Autodesk Inventor part; units mm, degrees
ref_plane "YZ Plane" through (0, 0, 0) normal (1, 0, 0) x (0, 1, 0)
ref_plane "XZ Plane" through (0, 0, 0) normal (0, 1, 0) x (-1, 0, 0)
ref_plane "XY Plane" through (0, 0, 0) normal (0, 0, 1) x (1, 0, 0)
sketch "Esboço1" plane through (0, 0, 0) normal (0, 1, 0) x (-1, 0, 0)
  circle A0 centre (0, 0) radius 9
  dimension "d0" = 18
extrude "Extrusão1" add sketch "Esboço1" along normal blind 5
sketch "Esboço2" plane through (0, 5, 0) normal (0, 1, 0) x (1, 0, 0)
  circle A0 centre (0, 0) radius 6
  dimension "d3" = 12
extrude "Extrusão2" add sketch "Esboço2" along normal blind 15
sketch "Esboço3" plane through (0, 20, 0) normal (0, 1, 0) x (1, 0, 0)
  point P0 (0, 0)
sketch "Esboço4" plane through (0, 20, 0) normal (0, 1, 0) x (1, 0, 0)
  circle A0 centre (0, 0) radius 4.275
  dimension "d6" = 8.55
extrude "Extrusão3" cut sketch "Esboço4" against normal through all
fillet "Arredondamento1" radius 2 1 edges at (-6, 5, 0)
properties part number "Espaçadores"
The model under review builds one solid part; all positions refer to its coordinate system, in mm. A direction names the side the tool comes from. Give positions to 0.01 mm unless a question says otherwise; leave off trailing zeros. Write each loop counter-clockwise with the first axis right and the second up, starting at its lowest first coordinate (ties: lowest second). Pieces come first, ordered by that corner, then holes. Notation, with made-up numbers: M 45.25,49 L 78.25,49 A19 cw 78.25,83 Z; hole C -36.75,-21.5 d3. An arc over 180 degrees is marked long. Write item = value, one per line. Start each with the question number.
Q1. For line 1 (Z direction, x = 0, y = 9.75) (3 decimals); line 2 (Z direction, x = 2, y = 15.25), list the stretches that pass through material, from the lowest coordinate up.
Q2. We need section C-C (y = 4.5). State the section outline as (x, z) points (3 decimals).
Q3. We need section A-A (z = 0). State the section outline as (x, y) points (3 decimals).
Q4. We need section B-B (x = 0). State the section outline as (y, z) points (3 decimals), plus the area to 3 significant figures.
Q5. Clearance check with flat-ended pins moving along their axes: pin 1 (4 mm diameter, centred on x = -5.5, y = 6, fed in from -Z); pin 2 (6 mm diameter, centred on y = 16, z = -6.5, fed in from -X); pin 3 (4 mm diameter, centred on x = -4, y = 6.5, fed in from +Z). State where each tip first meets the part, or that it passes through.
Q6. Mouldability with a two-part tool opening along X and no side actions: class faces 3 (the face through (1.172, 2.465, -8.923)), 4 (the face through (-2, 0, -4)), 5 (the face through (4.08, 10.14, -1.28)) as released by +X, released by -X, zero draft, split by the parting line, or undercut.
Q7. Machinability: for faces 1 (the face through (-6, 13, 0)), 2 (the face through (3, 20, 4)), which of the approach directions +Z, -Z, +X, -X, +Y, -Y give a long, thin tool a straight path to every point of the face, cutting with its end or side? Answer none if there is none.
Q8. We need section D-D (y = 9). State the section outline as (x, z) points (3 decimals), plus the area to 3 significant figures.
Result set:
q1.line_1 = -6 to -4.275, 4.275 to 6
q1.line_2 = -5.66 to -3.78, 3.78 to 5.66
q2.outline = C 0,0 d18; hole C 0,0 d8.55
q3.outline = M -9,0 L -4.275,0 L -4.275,20 L -6,20 L -6,7 A2 cw -8,5 L -9,5 Z; M 4.275,0 L 9,0 L 9,5 L 8,5 A2 cw 6,7 L 6,20 L 4.275,20 Z
q4.outline = M 0,-9 L 5,-9 L 5,-8 A2 cw 7,-6 L 20,-6 L 20,-4.275 L 0,-4.275 Z; M 0,4.275 L 20,4.275 L 20,6 L 7,6 A2 cw 5,8 L 5,9 L 0,9 Z
q4.area = 101 mm2
q5.pin_1 = -8.17
q5.pin_2 = -4.87
q5.pin_3 = 8.59
q6.face_3 = split by the parting line
q6.face_4 = zero draft
q6.face_5 = undercut
q7.face_1 = +Y
q7.face_2 = +Z, -Z, +X, -X, +Y
q8.outline = C 0,0 d12; hole C 0,0 d8.55
q8.area = 55.7 mm2
